The model under review builds one solid part; all positions refer to its coordinate system, in mm. Face numbers are marked on the shaded views. A direction names the side the tool comes from. Round coordinates to 2 decimals unless told otherwise and drop trailing zeros. Loops run counter-clockwise (first coordinate to the right, second up) from the corner with the lowest first, then second, coordinate; pieces in that order, holes last. Notation, with made-up numbers: M -30.5,14 L -13.5,14 A4 cw -13.5,19 Z; hole C -13.5,11.25 d1. An arc over 180 degrees is marked long. Answer as a JSON object with one key per item and string values. Group by question number.
Item 1: Consider section B-B (z = 3.5). Give the boundary of the cut face in (x, y).
Item 2: Consider section C-C (x = 4). Give the boundary of the cut face in (y, z), and give its area (3 significant figures).
Item 3: Insertion check: P1, Ø5, axis at x = -0.5, z = -4.5, coming from the -Y side. The pin has a flat end and moves straight along its axis. Give the tip position at first contact, or say it passes through.
Item 4: The part is to be moulded in two halves that separate along Z. For the marked faces 3, 4 and 5, say which applies: +Z half, -Z half, draft (parallel to the pull), parting line (faces both ways), or undercut.
Item 5: To check wall thickness, follow line 1 (X direction, y = 88.5, z = -3). State the ranges of the line that lie inside material, in increasing order.
Item 6: Consider section A-A (y = 94). Give the boundary of the cut face in (x, z), and give its area (3 significant figures).
Item 7: Tool access review of the marked faces 1 and 2: name each direction out of +Z, -Z, +X, -X, +Y, -Y from which nothing blocks a thin tool from reaching the whole face with its end or side.
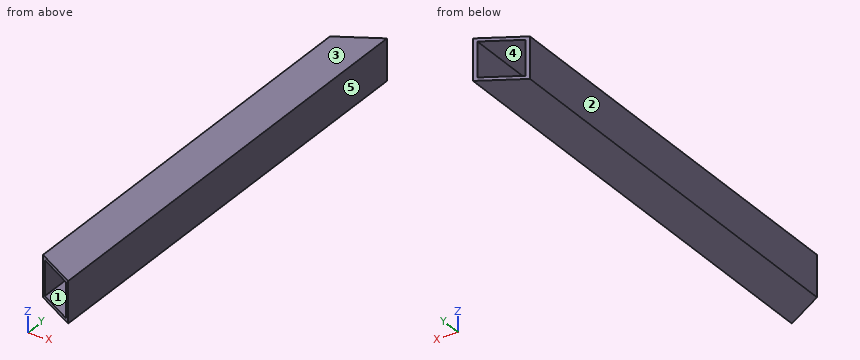
```python
from build123d import *

# Parameters (mm, degrees)
SKETCH1_W               = 13
SKETCH1_H               = 13
SKETCH1_W_2             = 11
SKETCH1_H_2             = 11
BOSS_EXTRUDE1_DEPTH     = 150
CUT_EXTRUDE1_DEPTH      = 1
CUT_EXTRUDE1_DEPTH_BACK = 14
SKETCH3_OUTSIDE_W       = 45.224
SKETCH3_OUTSIDE_H       = 182.224
CUT_EXTRUDE2_DEPTH      = 1
CUT_EXTRUDE2_DEPTH_BACK = 14


with BuildPart() as part:
    # Sketch1 → Boss-Extrude1 (new body)
    with BuildSketch(Plane(origin=(0, 0, 0), x_dir=(1, 0, 0), z_dir=(0, 1, 0))):
        Rectangle(SKETCH1_W, SKETCH1_H)
        Rectangle(SKETCH1_W_2, SKETCH1_H_2, mode=Mode.SUBTRACT)
    extrude(amount=BOSS_EXTRUDE1_DEPTH)

    # Sketch2 → Cut-Extrude1 (cut, two sides)
    with BuildSketch(Plane.XY.offset(6.5)) as cut_extrude1_sk:
        Polygon((275.941771788, 305.562279473), (6.5, 150), (-6.5, 142.494446501), (-275.941771788, -13.067832972), (-587.066330733, 525.815710604), (-35.182787157, 844.445823048), align=None)
    extrude(amount=CUT_EXTRUDE1_DEPTH, mode=Mode.SUBTRACT)
    extrude(cut_extrude1_sk.sketch, amount=-CUT_EXTRUDE1_DEPTH_BACK, mode=Mode.SUBTRACT)

    # Sketch3 outside → Cut-Extrude2 (cut, two sides)
    with BuildSketch(Plane.XY.offset(6.5)) as cut_extrude2_sk:
        with Locations((0, 75)):
            Rectangle(SKETCH3_OUTSIDE_W, SKETCH3_OUTSIDE_H)
        Polygon((6.5, 0), (-6.5, 7.505553499), (-6.5, 142.494446501), (6.5, 150), align=None, mode=Mode.SUBTRACT)
    extrude(amount=CUT_EXTRUDE2_DEPTH, mode=Mode.SUBTRACT)
    extrude(cut_extrude2_sk.sketch, amount=-CUT_EXTRUDE2_DEPTH_BACK, mode=Mode.SUBTRACT)


solid = part.part
```
Geometry results:
{
 "1": {"outline": "M -6.5,7.51 L -5.5,6.93 L -5.5,143.07 L -6.5,142.49 Z; M 5.5,0.58 L 6.5,0 L 6.5,150 L 5.5,149.42 Z"},
 "2": {"outline": "M 1.44,-6.5 L 148.56,-6.5 L 148.56,-5.5 L 1.44,-5.5 Z; M 1.44,5.5 L 148.56,5.5 L 148.56,6.5 L 1.44,6.5 Z", "area": "294 mm^2"},
 "3": {"P1": "stops at y = 2.72"},
 "4": {"face 3": "+Z half", "face 4": "undercut", "face 5": "draft"},
 "5": {"line 1": "x = -6.5 to -5.5, 5.5 to 6.5"},
 "6": {"outline": "M -6.5,-6.5 L 6.5,-6.5 L 6.5,6.5 L -6.5,6.5 Z; hole M -5.5,-5.5 L 5.5,-5.5 L 5.5,5.5 L -5.5,5.5 Z", "area": "48.0 mm^2"},
 "7": {"face 1": "+Y, -Y", "face 2": "+Z, -Z, -X, +Y, -Y"}
}
